from build123d import *

# Parameters (mm, degrees)
CYLINDER077_R     = 1.38
CYLINDER077_DEPTH = 13
CYLINDER076_R     = 1.38
CYLINDER076_DEPTH = 13
CYLINDER075_R     = 1.38
CYLINDER075_DEPTH = 13
BOX042_W          = 10
BOX042_H          = 145
BOX042_DEPTH      = 4
FILLET009_R       = 3


with BuildPart() as cylinder077:
    # Cylinder077 → Cylinder077 (new body)
    with BuildSketch(Plane(origin=(25, 188.5, 59), x_dir=(1, 0, 0), z_dir=(0, 0, 1))):
        Circle(CYLINDER077_R)
    extrude(amount=CYLINDER077_DEPTH)


with BuildPart() as cylinder076:
    # Cylinder076 → Cylinder076 (new body)
    with BuildSketch(Plane(origin=(25, 126.5, 59), x_dir=(1, 0, 0), z_dir=(0, 0, 1))):
        Circle(CYLINDER076_R)
    extrude(amount=CYLINDER076_DEPTH)


with BuildPart() as cylinder075:
    # Cylinder075 → Cylinder075 (new body)
    with BuildSketch(Plane(origin=(25, 64.5, 59), x_dir=(1, 0, 0), z_dir=(0, 0, 1))):
        Circle(CYLINDER075_R)
    extrude(amount=CYLINDER075_DEPTH)


with BuildPart() as obj1:
    # Box042 → Box042 (new body)
    with BuildSketch(Plane(origin=(20, 51, 66), x_dir=(1, 0, 0), z_dir=(0, 0, 1))):
        with Locations((5, 72.5)):
            Rectangle(BOX042_W, BOX042_H)
    extrude(amount=BOX042_DEPTH)

    # Fillet009
    fillet009_edges = [obj1.edges().sort_by_distance(p)[0] for p in [
        (20, 51, 68),
        (20, 196, 68),
        (30, 51, 68),
        (30, 196, 68),
    ]]
    fillet(fillet009_edges, radius=FILLET009_R)

    # Cut050: cut Cylinder075
    add(cylinder075.part, mode=Mode.SUBTRACT)

    # Cut051: cut Cylinder076
    add(cylinder076.part, mode=Mode.SUBTRACT)

    # Cut052: cut Cylinder077
    add(cylinder077.part, mode=Mode.SUBTRACT)


solid = obj1.part
Read the model definition and answer for the solid it produces. Units are mm, in the model's axes. Round coordinates to 2 decimals unless told otherwise and drop trailing zeros. Order: outer loops, then holes, each group sorted by start corner. A loop starts at its lowest first (then second) coordinate and runs counter-clockwise, first axis right, second up.
1) Straight lines are drawn through the part: L1, parallel to Y at x = 25, z = 68.25; L2, parallel to X at y = 188.5, z = 69.1; L3, parallel to Y at x = 26, z = 66.5. For each, find the intervals that lie inside material, in ascending order.
2) The part is cut by section C-C on x = 25. Write down the section's boundary in (y, z), plus the area to 3 significant figures.
3) The part is cut by section B-B on z = 67.35. Write down the section's boundary in (x, y).
4) The part is cut by section A-A on y = 64.5. Write down the section's boundary in (x, z), plus the area to 3 significant figures.
5) The mould has two halves that part along Y. Classify faces 1 (the face through (25, 51, 68)), 2 (the face through (24.9, 124.5, 66)), 3 (the face through (24.82, 189.87, 67.97)): released by +Y, released by -Y, zero draft, split by the parting line, or undercut.
Resolved:
1. L1: y = 51 to 63.12, 65.88 to 125.12, 127.88 to 187.12, 189.88 to 196
1. L2: x = 20 to 23.62, 26.38 to 30
1. L3: y = 51 to 63.55, 65.45 to 125.55, 127.45 to 187.55, 189.45 to 196
2. outline: (51, 66) - (63.12, 66) - (63.12, 70) - (51, 70) - close; (65.88, 66) - (125.12, 66) - (125.12, 70) - (65.88, 70) - close; (127.88, 66) - (187.12, 66) - (187.12, 70) - (127.88, 70) - close; (189.88, 66) - (196, 66) - (196, 70) - (189.88, 70) - close
2. area: 547 mm2
3. outline: (20, 54) arc R3 ccw to (23, 51) - (27, 51) arc R3 ccw to (30, 54) - (30, 193) arc R3 ccw to (27, 196) - (23, 196) arc R3 ccw to (20, 193) - close; hole circle Ø2.76 at (25, 64.5); hole circle Ø2.76 at (25, 126.5); hole circle Ø2.76 at (25, 188.5)
4. outline: (20, 66) - (23.62, 66) - (23.62, 70) - (20, 70) - close; (26.38, 66) - (30, 66) - (30, 70) - (26.38, 70) - close
4. area: 29.0 mm2
5. face 1: released by -Y
5. face 2: zero draft
5. face 3: undercut
